The model under review builds one solid part; all positions refer to its coordinate system, in mm. Face numbers are marked on the shaded views. A direction names the side the tool comes from. Round coordinates to 2 decimals unless told otherwise and drop trailing zeros. Loops run counter-clockwise (first coordinate to the right, second up) from the corner with the lowest first, then second, coordinate; pieces in that order, holes last. Notation, with made-up numbers: (-18.75, -32.5) -> (-3.75, -32.5) arc R31 ccw to (-3.75, 3.5) -> close; hole circle Ø4 at (12.5, -32.75). An arc over 180 degrees is marked (long way). Use a Markdown table: item, result. Add a question column.
1) Consider section C-C on y = 12.5. Give the boundary of the cut face in (x, z).
2) For the marked faces 1, 2 and 3, list the 3-axis set-ups (+Z, -Z, +X, -X, +Y, -Y) from which the entire face can be reached by the end or side of a thin tool; tool diameter is ignored.
3) Consider section A-A on z = -2.5. Give the boundary of the cut face in (x, y).
4) Consider section B-B on x = -66. Give the boundary of the cut face in (y, z), plus the area to 3 significant figures.
5) Wall thickness on probe 1 along X at (y, z) = (14, -12.5); probe 2 along X at (y, z) = (14, -4.5); probe 3 along X at (y, z) = (17.5, -14): over which ranges is each line inside the solid? List them lowest first.
6) Mouldability with a two-part tool opening along Y and no side actions: class the marked faces 4, 5 and 6 as released by +Y, released by -Y, zero draft, split by the parting line, or undercut.
7) Insertion check: pin 1 (4 mm diameter, centred on y = 10.5, z = 10, fed in from +X); pin 2 (5 mm diameter, centred on x = -47.5, z = -2, fed in from +Y); pin 3 (2 mm diameter, centred on x = -60.5, z = -14, fed in from +Y). Each pin has a flat end and moves straight along its axis. Give the tip position at first contact, or say it passes through.
8) Consider section D-D on z = 12.5. Give the boundary of the cut face in (x, y), plus the area to 3 significant figures.
from build123d import *

# Parameters (mm, degrees)
EXTRUDE_THIN1_DEPTH              = 19.05
SKETCH8_W                        = 25.4
SKETCH8_H                        = 38.1
BOSS_EXTRUDE1_DEPTH              = 19.05
CUT_EXTRUDE3_DEPTH               = 87.66947312
CUT_EXTRUDE3_DEPTH_BACK          = 87.66947312
CUT_EXTRUDE4_REACH               = 76.686
CUT_EXTRUDE4_OFFSET_FROM_SURFACE = 2.54
SKETCH13_W                       = 12.954
SKETCH13_H                       = 12.954
CUT_EXTRUDE4_DIRECTION_2_DEPTH   = 73.146238944


with BuildPart() as part:
    # Sketch1 → Extrude-Thin1 (new, symmetric)
    with BuildSketch(Plane.XY):
        Polygon((-56.518566399, -10.196160483), (-71.084509945, 0), (-55.790269221, 21.84891532), (-24.57753305, 0), (-26.034127404, -2.080849078), (-55.166014498, 18.311471887), (-67.547066513, 0.624254723), (-55.061972044, -8.115311405), align=None)
    extrude(amount=EXTRUDE_THIN1_DEPTH, both=True)

    # Sketch8 → Boss-Extrude1 (add)
    with BuildSketch(Plane(origin=(-16.494988624, 11.546492037, 0), x_dir=(0.5734623443633238, 0.8192319205190437, 0), z_dir=(0.8192319205190437, -0.5734623443633238, 0))):
        with Locations((-1.394289721, 0)):
            Rectangle(SKETCH8_W, SKETCH8_H)
    extrude(amount=-BOSS_EXTRUDE1_DEPTH)

    # Sketch12 → Cut-Extrude3 (cut, two sides: drawn at the far end of the back side and taken through both)
    with BuildSketch(Plane(origin=(0, 0, -19.05), x_dir=(-1, 0, 0), z_dir=(0, 0, -1)).offset(-CUT_EXTRUDE3_DEPTH_BACK)):
        Polygon((40.183901135, 10.92445766), (12.895806765, 22.827442865), (25.617957589, 31.732948441), align=None)
    extrude(amount=CUT_EXTRUDE3_DEPTH + CUT_EXTRUDE3_DEPTH_BACK, mode=Mode.SUBTRACT)

    # Cut-Extrude4: up to this face of the body (flat: up to its plane, moved by the offset)
    cut_extrude4_end = Plane(part.part.faces().sort_by_distance((-40.600070951, 8.115311405, 0))[0]).offset(-CUT_EXTRUDE4_OFFSET_FROM_SURFACE)
    # Sketch13 → Cut-Extrude4 (cut, up to the picked face)
    with BuildSketch(Plane(origin=(-10.426997364, 23.904330147, 0), x_dir=(0.9165953540643084, 0.3998161538854141, 0), z_dir=(-0.3998161538854141, 0.9165953540643084, 0)), mode=Mode.PRIVATE) as cut_extrude4_sk1:
        with Locations((-17.579029301, 0)):
            Rectangle(SKETCH13_W, SKETCH13_H)
    cut_extrude4_tool1 = split(extrude(cut_extrude4_sk1.sketch, amount=-CUT_EXTRUDE4_REACH, mode=Mode.PRIVATE), bisect_by=cut_extrude4_end, keep=Keep.BOTH, mode=Mode.PRIVATE)
    add(cut_extrude4_tool1.solids().sort_by(Axis((-26.539854, 16.87595, 0), (0.3998161538854141, -0.9165953540643084, 0)))[0], mode=Mode.SUBTRACT)

    # Sketch13 → Cut-Extrude4 direction 2 (cut)
    with BuildSketch(Plane(origin=(-10.426997364, 23.904330147, 0), x_dir=(0.9165953540643084, 0.3998161538854141, 0), z_dir=(-0.3998161538854141, 0.9165953540643084, 0))):
        with Locations((-17.579029301, 0)):
            Rectangle(SKETCH13_W, SKETCH13_H)
    extrude(amount=CUT_EXTRUDE4_DIRECTION_2_DEPTH, mode=Mode.SUBTRACT)


solid = part.part
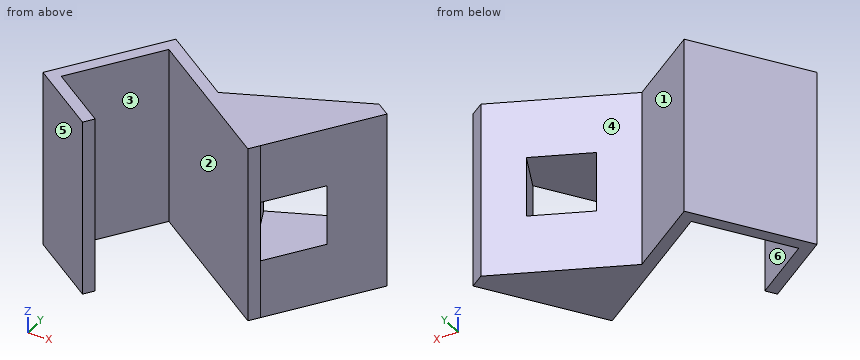
Result set:
| question | item | result |
|---|---|---|
| 1 | outline | (-62.33, -19.05) -> (-59.23, -19.05) -> (-59.23, 19.05) -> (-62.33, 19.05) -> close; (-46.86, -19.05) -> (-42.43, -19.05) -> (-42.43, 19.05) -> (-46.86, 19.05) -> close; (-36.57, -19.05) -> (-15.83, -19.05) -> (-15.83, 19.05) -> (-36.57, 19.05) -> close; hole (-31.7, -6.48) -> (-17.56, -6.48) -> (-17.56, 6.48) -> (-31.7, 6.48) -> close |
| 2 | face 1 | +Z, -Z, +Y |
| 2 | face 2 | +Z, -Z, -Y |
| 2 | face 3 | +Z, -Z |
| 3 | outline | (-71.08, 0) -> (-56.52, -10.2) -> (-55.06, -8.12) -> (-67.55, 0.62) -> (-55.17, 18.31) -> (-26.03, -2.08) -> (-24.58, 0) -> (-26.98, 1.68) -> (-32.48, 14.29) -> (-40.18, 10.92) -> (-55.79, 21.85) -> close; (-20.6, 19.47) -> (-16.9, 10.97) -> (-10.01, 20.81) -> (-12.9, 22.83) -> close |
| 4 | outline | (-3.56, -19.05) -> (-0.46, -19.05) -> (-0.46, 19.05) -> (-3.56, 19.05) -> close; (2.83, -19.05) -> (7.26, -19.05) -> (7.26, 19.05) -> (2.83, 19.05) -> close |
| 4 | area | 287 mm2 |
| 5 | probe 1 | -61.28 to -58.18, -49.01 to -44.58, -33.13 to -14.78 |
| 5 | probe 2 | -61.28 to -58.18, -49.01 to -44.58, -33.13 to -32.35, -18.22 to -14.78 |
| 5 | probe 3 | -58.83 to -55.73, -54.01 to -49.58, -25.11 to -12.33 |
| 6 | face 4 | released by +Y |
| 6 | face 5 | released by -Y |
| 6 | face 6 | undercut |
| 7 | pin 1 | x = -15.83 |
| 7 | pin 2 | y = 17.8 |
| 7 | pin 3 | y = 16.55 |
| 8 | outline | (-71.08, 0) -> (-56.52, -10.2) -> (-55.06, -8.12) -> (-67.55, 0.62) -> (-55.17, 18.31) -> (-26.03, -2.08) -> (-10.01, 20.81) -> (-12.9, 22.83) -> (-40.18, 10.92) -> (-55.79, 21.85) -> close |
| 8 | area | 483 mm2 |
